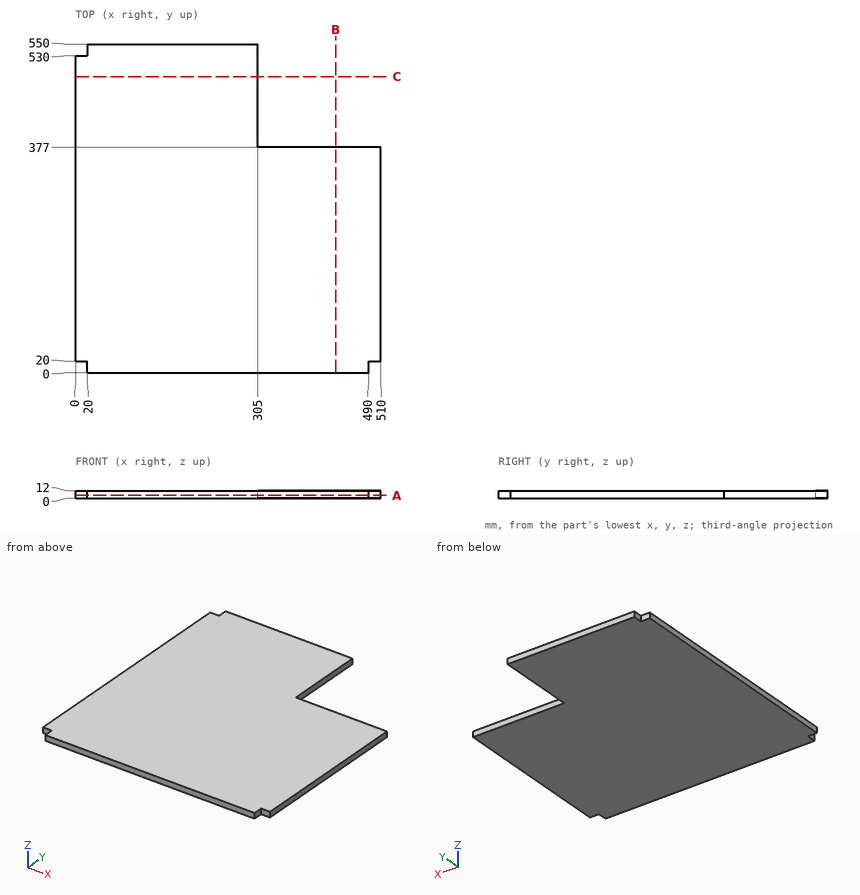
Input: dimensioned drawing with shaded views. Units: mm. Origin: part minimum x, y, z. Coordinates: 2 decimals unless noted, no trailing zeros. Order: outer loops, then holes, each group sorted by start corner. A loop starts at its lowest first (then second) coordinate and runs counter-clockwise, first axis right, second up.
(1) Material intervals for probe 1 along Y at (x, z) = (467, 11), sorted ascending.
(2) First-contact query: pin 1 (3.5 mm diameter, centred on y = 13.5, z = 3.5, fed in from +X); pin 2 (3.5 mm diameter, centred on x = 11.5, z = 4, fed in from -Y); pin 3 (3.5 mm diameter, centred on y = 545, z = 6.5, fed in from -X). Flat tips, straight axial feed; report the tip coordinate or a pass-through.
(3) Section query A-A (z = 4.5). Return the cut outline in (x, y).
(4) Section query B-B (x = 435). Return the cut outline in (y, z), plus the area to 3 significant figures.
(5) Section query C-C (y = 495.5). Return the cut outline in (x, z), plus the area to 3 significant figures.
Solution:
1. probe 1: y = 0 to 377
2. pin 1: stops at x = 490
2. pin 2: stops at y = 20
2. pin 3: stops at x = 20
3. outline: (0, 20) - (20, 20) - (20, 0) - (490, 0) - (490, 20) - (510, 20) - (510, 377) - (305, 377) - (305, 550) - (20, 550) - (20, 530) - (0, 530) - close
4. outline: (0, 0) - (377, 0) - (377, 12) - (0, 12) - close
4. area: 4,520 mm2
5. outline: (0, 0) - (305, 0) - (305, 12) - (0, 12) - close
5. area: 3,660 mm2
